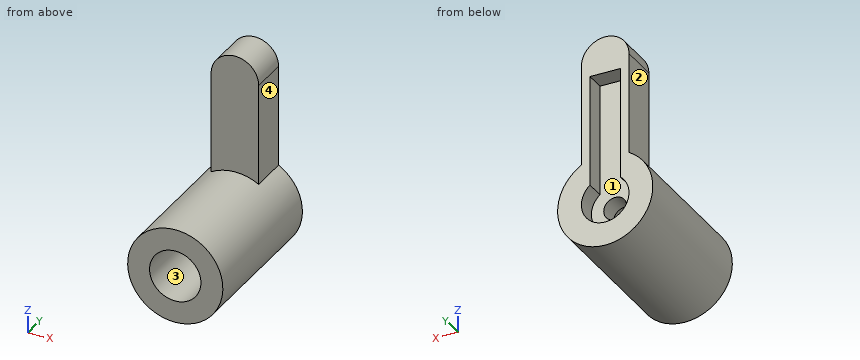
```python
from build123d import *

# Parameters (mm, degrees)
SKETCH1_R           = 1.524
BOSS_EXTRUDE1_DEPTH = 5.08
SKETCH2_R           = 3.175
SKETCH2_W           = 4.064
SKETCH2_H           = 17.78
CUT_EXTRUDE1_DEPTH  = 2.54
BOSS_EXTRUDE2_START = 15.24
SKETCH3_R           = 6.35
BOSS_EXTRUDE2_DEPTH = 15.24
SKETCH4_R           = 3.429
CUT_EXTRUDE2_DEPTH  = 15.24


with BuildPart() as part:
    # Sketch1 → Boss-Extrude1 (new body)
    with BuildSketch(Plane(origin=(0, 0, 0), x_dir=(1, 0, 0), z_dir=(0, 1, 0))):
        with BuildLine():
            ThreePointArc((3.175, -5.499261314), (0, 6.35), (-3.175, -5.499261314))
            Line((-3.175, -5.499261314), (-3.175, -19.05))
            ThreePointArc((-3.175, -19.05), (0, -22.225), (3.175, -19.05))
            Line((3.175, -19.05), (3.175, -5.499261314))
        make_face()
        with Locations(Location((0, 0, 0), (0, 0, 270))):
            Circle(SKETCH1_R, mode=Mode.SUBTRACT)
    extrude(amount=BOSS_EXTRUDE1_DEPTH)

    # Sketch2 → Cut-Extrude1 (cut)
    with BuildSketch(Plane(origin=(0, 5.08, 0), x_dir=(1, 0, 0), z_dir=(0, 1, 0))):
        Circle(SKETCH2_R)
        with Locations((0, -8.434547342)):
            Rectangle(SKETCH2_W, SKETCH2_H)
    extrude(amount=-CUT_EXTRUDE1_DEPTH, mode=Mode.SUBTRACT)

    # Sketch3 → Boss-Extrude2 (add)
    with BuildSketch(Plane.XZ.offset(BOSS_EXTRUDE2_START)):
        with Locations(Location((0, 0, 0), (0, 0, 270))):
            Circle(SKETCH3_R)
    extrude(amount=-BOSS_EXTRUDE2_DEPTH)

    # Sketch4 → Cut-Extrude2 (cut)
    with BuildSketch(Plane.XZ.offset(15.24)):
        with Locations(Location((0, 0, 0), (0, 0, 270))):
            Circle(SKETCH4_R)
    extrude(amount=-CUT_EXTRUDE2_DEPTH, mode=Mode.SUBTRACT)


solid = part.part
```
Verification items for the finished model (mm, model axes). Face numbers are marked on the shaded views. Give positions to 0.01 mm unless a question says otherwise; leave off trailing zeros. Order: outer loops, then holes, each group sorted by start corner. A loop starts at its lowest first (then second) coordinate and runs counter-clockwise, first axis right, second up. Notation, with made-up numbers: M -7.5,59 L 34.5,59 A27 ccw 34.5,87 Z; hole C 63.5,-22.5 d8. An arc over 180 degrees is marked long. Return JSON: item names as keys, results as strings. Group by question number.
1) Section check C-C on y = 3.5. Record the cut outline in (x, z) (3 decimals).
2) Section check A-A on z = 0. Record the cut outline in (x, y) (3 decimals), and give its area (3 significant figures).
3) Scan lines: line 1 (X direction, y = -11.5, z = 0); line 2 (Y direction, x = 0.5, z = 9.5); line 3 (X direction, y = 3.1, z = 0) (3 decimals). Record each from-to range of solid material in increasing order.
4) Go/stop test with flat-tipped pins: pin 1 Ø4 at (x, z) = (0, 0) entering from +Y; pin 2 Ø4 at (y, z) = (2.5, 9.5) entering from -X (3 decimals); pin 3 Ø3 at (x, z) = (-3.5, 12.5) entering from -Y; pin 4 Ø1.8 at (x, z) = (0, 0) entering from -Y. Record where each tip stops, or that it passes through.
5) Section check D-D on z = 8. Record the cut outline in (x, y) (3 decimals), and give its area (3 significant figures).
6) Mould release check, pull along X, two halves, no side actions. Record for the marked faces 1, 2, 3 and 4: pulls with the +X half, pulls with the -X half, needs draft (parallel to the pull), parting line crosses it, or undercut.
7) Section check B-B on x = 0. Record the cut outline in (y, z) (3 decimals).
Answer block:
{
 "1": {"outline": "M -3.175,5.499 A6.35 ccw long 3.175,5.499 L 3.175,19.05 A3.175 ccw -3.175,19.05 Z; hole M -2.032,2.44 A3.175 ccw long 2.032,2.44 L 2.032,17.325 L -2.032,17.325 Z"},
 "2": {"outline": "M -6.35,-15.24 L -3.429,-15.24 L -3.429,0 L -1.524,0 L -1.524,2.54 L -3.175,2.54 L -3.175,5.08 L -6.35,5.08 Z; M 1.524,0 L 3.429,0 L 3.429,-15.24 L 6.35,-15.24 L 6.35,5.08 L 3.175,5.08 L 3.175,2.54 L 1.524,2.54 Z", "area": "130 mm^2"},
 "3": {"line 1": "x = -6.35 to -3.43, 3.43 to 6.35", "line 2": "y = 0 to 2.54", "line 3": "x = -6.35 to -3.175, 3.175 to 6.35"},
 "4": {"pin 1": "stops at y = 2.54", "pin 2": "stops at x = -3.175", "pin 3": "stops at y = 0", "pin 4": "passes through"},
 "5": {"outline": "M -3.175,0 L 3.175,0 L 3.175,5.08 L 2.032,5.08 L 2.032,2.54 L -2.032,2.54 L -2.032,5.08 L -3.175,5.08 Z", "area": "21.9 mm^2"},
 "6": {"face 1": "undercut", "face 2": "pulls with the -X half", "face 3": "undercut", "face 4": "pulls with the +X half"},
 "7": {"outline": "M -15.24,-6.35 L 5.08,-6.35 L 5.08,-3.175 L 2.54,-3.175 L 2.54,-1.524 L 0,-1.524 L 0,-3.429 L -15.24,-3.429 Z; M -15.24,3.429 L 0,3.429 L 0,1.524 L 2.54,1.524 L 2.54,17.325 L 5.08,17.325 L 5.08,22.225 L 0,22.225 L 0,6.35 L -15.24,6.35 Z"}
}
